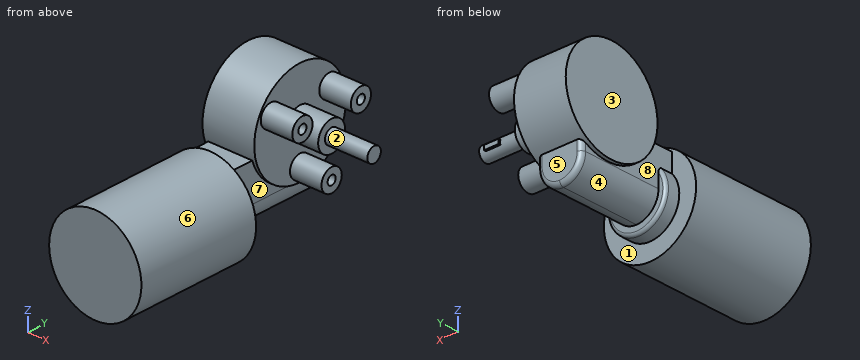
Autodesk Inventor part; units mm, degrees
ref_plane "Work Plane1" through (-31.5, 0, 0) normal (1, 0, 0) x (0, 1, 0)
ref_plane "Work Plane3" through (0, 0, -31.5) normal (0, 0, 1) x (1, 0, 0)
ref_plane "XZ Plane" through (0, 0, 0) normal (0, 1, 0) x (-1, 0, 0)
sketch "Sketch1" plane through (0, 0, 0) normal (0, 1, 0) x (-1, 0, 0)
  circle A0 centre (0, 0) radius 31.5
  circle A1 centre (0, 0) radius 20
  dimension "d0" = 63
  dimension "d29" = 40
extrude "Extrusion1" add sketch "Sketch1" along normal blind 85 contours A0 | A1
sketch "Sketch2" plane through (0, 0, 0) normal (1, 0, 0) x (0, 1, 0)
  line L0 (0, -31.5) -> (85, -31.5)
  line L1 (0, -31.5) -> (0, 69.5)
  line L2 (0, 69.5) -> (166.6, 69.5)
  line L3 (166.6, 69.5) -> (166.6, 35.5)
  line L4 (166.6, 35.5) -> (132.6, 35.5)
  circle A0 centre (132.6, 35.5) radius 34
  circle A1 centre (132.6, 35.5) radius 25
  circle A2 centre (132.6, 10.5) radius 7.5
  circle A3 centre (132.6, 10.5) radius 3
  circle A4 centre (154.2506, 48) radius 7.5
  circle A5 centre (154.2506, 48) radius 3
  circle A6 centre (110.9494, 48) radius 7.5
  circle A7 centre (110.9494, 48) radius 3
  line L5 (85, -31.5) -> (85, 31.5)
  line L6 (85, 25.7084) -> (151.9419, 25.7084)
  line L7 (151.9419, 25.7084) -> (151.9419, -14.2916)
  line L8 (151.9419, -14.2916) -> (85, -14.2916)
  line L9 (85, -14.2916) -> (85, 25.7084)
  circle A8 centre (132.6, 35.5) radius 10
  circle A9 centre (132.6, 35.5) radius 5
  line L10 (85, 31.5) -> (85, 0)
  line L11 (85, 0) -> (100.814, 0)
  point P0 (0, 0)
  point P1 (151.9419, 7.5377)
  point P2 (134.9384, 1.5805)
  point P3 (132.6, 1.5)
  point P4 (100.0404, 25.7084)
  point P5 (92.907, 0)
  dimension "d8" = 50
  dimension "d3" = 101
  dimension "d4" = 166.6
  dimension "d5" = 34
  dimension "d6" = 34
  dimension "d7" = 68
  dimension "d9" = 15
  dimension "d10" = 6
  dimension "d13" = 360
  dimension "d21" = 20
  dimension "d22" = 10
  dimension "d26" = 40
  dimension "d49" = 69.5
  dimension "d50" = 35.5
extrude "Extrusion2" add sketch "Sketch2" along normal mid plane 30 contours L5 L6 A0 L7 L8 | A0 L4 A1 A4 A6 L6 | A0 L7 A1 L4 | L6 A1 A2 L7 A0 | A1 L7 L6 A8 L4 | L4 A8 L6 A1 A6 A4 | L6 A8 L7 A1 A2 | A8 L6 | A4 A1 A5 | A1 A5 A4 | A6 A1 A7 | A1 A7 A6 | L6 A8 | A5 A1 | A1 A5 | A7 A1 | A1 A7 | A9
extrude "Extrusion3" add sketch "Sketch2" along normal blind 39.2 contours A8 L6 | A4 A1 A5 | A1 A5 A4 | A6 A1 A7 | A1 A7 A6 | A2 A1 A3 | A1 A3 A2 | L6 A8 | A5 A1 | A1 A5 | A7 A1 | A1 A7 | A3 A1 | A1 A3 | A9
extrude "Extrusion4" add sketch "Sketch2" along normal mid plane 35.35 contours A0 L4 A1 A4 A6 L6 | A0 L7 A1 L4 | L6 A1 A2 L7 A0 | A1 L7 L6 A8 L4 | L4 A8 L6 A1 A6 A4 | L6 A8 L7 A1 A2 | A8 L6 | A4 A1 A5 | A1 A5 A4 | A6 A1 A7 | A1 A7 A6 | A2 A1 A3 | A1 A3 A2 | L6 A8 | A5 A1 | A1 A5 | A7 A1 | A1 A7 | A3 A1 | A1 A3 | A9
extrude "Extrusion5" add sketch "Sketch2" along normal blind 68.2 contours A9
ref_plane "Work Plane1" through (-31.5, 0, 0) normal (1, 0, 0) x (0, 1, 0)
fillet "Fillet1" radius 15 2 edges at (15, 118.471, -14.2916) (-15, 118.471, -14.2916)
fillet "Fillet2" radius 3 3 edges at (15, 151.9419, 4.123) (-15, 151.9419, 4.123) (10.6066, 151.9419, -9.8982)
extrude "Extrusion6" add sketch "Sketch1" along normal blind 95 contours A1
fillet "Fillet3" radius 2 1 edges at (0, 95, -20)
ref_plane "Work Plane2" through (63.8, 132.6, 35.5) normal (1, 0, 0) x (0, 0, -1)
sketch "Sketch3" plane through (39.2, 154.2506, 48) normal (1, 0, 0) x (0, 0, -1)
  circle A0 centre (0, 0) radius 3
  circle A1 centre (37.5, -21.6506) radius 7.5
  circle A2 centre (37.5, -21.6506) radius 3
  circle A3 centre (0, -43.3013) radius 7.5
  circle A4 centre (0, -43.3013) radius 3
  point P0 (48, -154.2506)
  dimension "d33" = 6
  dimension "d34" = 6
  dimension "d35" = 6
hole "Hole1" at (39.2, 154.2506, 48) at (39.2, 132.6, 10.5) at (39.2, 110.9494, 48) direction (-1, 0, 0) diameter 6 depth 10
sketch "Sketch4" plane through (63.8, 132.6, 35.5) normal (1, 0, 0) x (0, 0, -1)
  line L0 (-1.5, 3.8) -> (1.5, 3.8)
  line L1 (1.5, 3.8) -> (1.5, 6.2)
  line L2 (1.5, 6.2) -> (-1.5, 6.2)
  line L3 (-1.5, 6.2) -> (-1.5, 3.8)
  circle A0 centre (0, 0) radius 5
  line L4 (-1.5, 3.8) -> (1.5, 6.2) construction
  line L5 (1.5, 3.8) -> (-1.5, 6.2) construction
  point P0 (35.5, -132.6)
  point P1 (0, 5)
  point P2 (-1.5, 4.7697)
  point P3 (1.5, 4.7697)
  dimension "d43" = 1.2
  dimension "d44" = 3
extrude "Extrusion7" add sketch "Sketch4" against normal blind 9.9 contours L3 L2 L1 A0
ref_plane "Work Plane3" through (0, 0, -31.5) normal (0, 0, 1) x (1, 0, 0)
properties part number "motor" material "ABS Plastic"
Verification items for the finished model (mm, model axes). Face numbers are marked on the shaded views. A direction names the side the tool comes from. Give positions to 0.01 mm unless a question says otherwise; leave off trailing zeros. Order: outer loops, then holes, each group sorted by start corner. A loop starts at its lowest first (then second) coordinate and runs counter-clockwise, first axis right, second up. Notation, with made-up numbers: (61, 29.25) - (73, 29.25) arc R10 ccw to (73, 41.25) - close; hole circle Ø11 at (72.5, 71). An arc over 180 degrees is marked (long way). Answer as CSV lines item,"result". Start each with the question number.
Item 1: Section check D-D, the plane y = 20.5. Record the boundary of the cut face in (x, z).
Item 2: Gauge pin test, flat ends, axial feed: pin 1 (8 mm diameter, centred on y = 154.25, z = 48, fed in from -X) (3 decimals); pin 2 (7 mm diameter, centred on y = 110.95, z = 48, fed in from +X); pin 3 (3 mm diameter, centred on y = 119.5, z = -8.5, fed in from -X). Record the tip position at first contact, or that the pin passes through.
Item 3: Access from +Z, -Z, +X, -X, +Y, -Y to the whole of each face (thin tool, end or side, straight path). Record for the marked faces 4, 5, 6, 7 and 8.
Item 4: Section check B-B, the plane z = 48. Record the boundary of the cut face in (x, y) (3 decimals).
Item 5: Mould release check, pull along Y, two halves, no side actions. Record for the marked faces 1, 2 and 3: released by +Y, released by -Y, zero draft, split by the parting line, or undercut.
Item 6: Section check C-C, the plane x = -25. Record the boundary of the cut face in (y, z), plus the area to 3 significant figures.
Item 7: Material ranges on L1, parallel to Z at x = 34.75, y = 132.6; L2, parallel to Y at x = 33, z = 10; L3, parallel to Y at x = 33.75, z = 48, recorded low to high.
Filled in:
1,outline,"circle Ø63 at (0, 0)"
2,pin 1,"x = -17.675"
2,pin 2,"x = 39.2"
2,pin 3,"x = -12.87"
3,face 4,"-Z, -X, +Y"
3,face 5,"-Z, +X, -X, +Y"
3,face 6,"-Y"
3,face 7,"+X"
3,face 8,"-X"
4,outline,"(-17.675, 100.981) - (17.675, 100.981) - (17.675, 103.449) - (39.2, 103.449) - (39.2, 107.949) - (29.2, 107.949) - (29.2, 113.949) - (39.2, 113.949) - (39.2, 118.449) - (17.675, 118.449) - (17.675, 146.751) - (39.2, 146.751) - (39.2, 151.251) - (29.2, 151.251) - (29.2, 157.251) - (39.2, 157.251) - (39.2, 161.751) - (17.675, 161.751) - (17.675, 164.219) - (-17.675, 164.219) - close"
5,face 1,"undercut"
5,face 2,"split by the parting line"
5,face 3,"zero draft"
6,outline,"(0, -19.16) - (85, -19.16) - (85, 19.16) - (0, 19.16) - close"
6,area,"3,260 mm^2"
7,L1,"3 to 7.5, 13.5 to 18, 25.5 to 45.5"
7,L2,"125.12 to 129.64, 135.56 to 140.08"
7,L3,"103.45 to 107.95, 113.95 to 118.45, 146.75 to 151.25, 157.25 to 161.75"
